Design review of the part built by this model. Coordinates are the model's own, in mm. Face numbers are marked on the shaded views. A direction names the side the tool comes from. Give positions to 0.01 mm unless a question says otherwise; leave off trailing zeros. Loops run counter-clockwise (first coordinate to the right, second up) from the corner with the lowest first, then second, coordinate; pieces in that order, holes last. Notation, with made-up numbers: (83.5, -5) -> (112.5, -5) arc R21 cw to (112.5, 19) -> close; hole circle Ø3 at (48, -25). An arc over 180 degrees is marked (long way). Use a Markdown table: item, result. Add a question column.
1. Add section B-B (y = 0). State the section outline as (x, z) points.
2. Add section A-A (z = 0). State the section outline as (x, y) points.
3. For pin 1 Ø6 at (y, z) = (0, 0) entering from +X; pin 2 Ø2 at (x, z) = (18, -22) entering from -Y, all flat-tipped, find the tip position at first contact; note any pin that passes through.
4. Add section D-D (y = 21). State the section outline as (x, z) points.
5. For the marked faces 1 and 2, list the 3-axis set-ups (+Z, -Z, +X, -X, +Y, -Y) from which the entire face can be reached by the end or side of a thin tool; tool diameter is ignored.
6. Add section C-C (z = -42.5). State the section outline as (x, y) points, and give its area (3 significant figures).
7. To check wall thickness, follow line 1 (Y direction, x = 1.1, z = 0); line 2 (X direction, y = 5.5, z = 30); line 3 (Y direction, x = 15.75, z = -27). State the ranges of each line that lie inside material, in increasing order.
```python
from build123d import *

# Parameters (mm, degrees)
SKETCH1_W           = 100
SKETCH1_H           = 65
SKETCH1_R           = 2.5
BOSS_EXTRUDE1_DEPTH = 2
SKETCH2_W           = 100
SKETCH2_H           = 5
BOSS_EXTRUDE2_DEPTH = 28


with BuildPart() as part:
    # Sketch1 → Boss-Extrude1 (new body)
    with BuildSketch(Plane(origin=(0, 0, 0), x_dir=(0, 0, -1), z_dir=(1, 0, 0))):
        Rectangle(SKETCH1_W, SKETCH1_H)
        Circle(SKETCH1_R, mode=Mode.SUBTRACT)
    extrude(amount=BOSS_EXTRUDE1_DEPTH)

    # Sketch2 → Boss-Extrude2 (add)
    with BuildSketch(Plane(origin=(2, 0, 0), x_dir=(0, 0, -1), z_dir=(1, 0, 0))):
        with Locations((0, 30)):
            Rectangle(SKETCH2_W, SKETCH2_H)
    extrude(amount=BOSS_EXTRUDE2_DEPTH)


solid = part.part
```
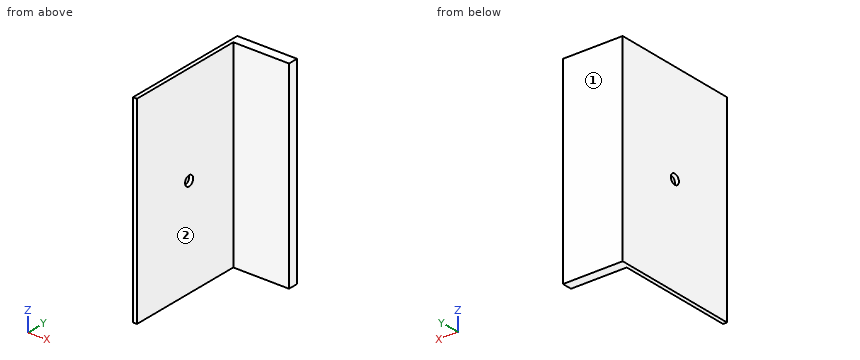
Taken from the geometry:
| question | item | result |
|---|---|---|
| 1 | outline | (0, -50) -> (2, -50) -> (2, -2.5) -> (0, -2.5) -> close; (0, 2.5) -> (2, 2.5) -> (2, 50) -> (0, 50) -> close |
| 2 | outline | (0, -32.5) -> (2, -32.5) -> (2, -2.5) -> (0, -2.5) -> close; (0, 2.5) -> (2, 2.5) -> (2, 27.5) -> (30, 27.5) -> (30, 32.5) -> (0, 32.5) -> close |
| 3 | pin 1 | stops at x = 2 |
| 3 | pin 2 | stops at y = 27.5 |
| 4 | outline | (0, -50) -> (2, -50) -> (2, 50) -> (0, 50) -> close |
| 5 | face 1 | +Z, -Z, +X, -X, +Y |
| 5 | face 2 | +Z, -Z, +X, -Y |
| 6 | outline | (0, -32.5) -> (2, -32.5) -> (2, 27.5) -> (30, 27.5) -> (30, 32.5) -> (0, 32.5) -> close |
| 6 | area | 270 mm^2 |
| 7 | line 1 | y = -32.5 to -2.5, 2.5 to 32.5 |
| 7 | line 2 | x = 0 to 2 |
| 7 | line 3 | y = 27.5 to 32.5 |
